The model under review builds one solid part; all positions refer to its coordinate system, in mm. A direction names the side the tool comes from. Round coordinates to 2 decimals unless told otherwise and drop trailing zeros. Order: outer loops, then holes, each group sorted by start corner. A loop starts at its lowest first (then second) coordinate and runs counter-clockwise, first axis right, second up. Notation, with made-up numbers: M -15,73.5 L 44,73.5 A17 ccw 44,80.5 Z; hole C 37,0.5 d11. An arc over 180 degrees is marked long. Use a Markdown table: item, result. Add a question column.
1. The part is to be moulded in two halves that separate along Z. For faces 1 (the flat face through (13, 4, 0)), 2 (the flat face through (0, 5, -12)), 3 (the cylindrical face through (3.451, 3.595, -13.421)), say which applies: +Z half, -Z half, draft (parallel to the pull), parting line (faces both ways), or undercut.
2. Consider section B-B on x = 2.25. State the section outline as (y, z) points.
3. Consider section C-C on y = 5.5. State the section outline as (x, z) points.
4. Insertion check: P1, Ø4, axis at x = 12, y = 4, coming from the -Z side; P2, Ø4, axis at y = 2.75, z = -12.5, coming from the +X side. Each pin has a flat end and moves straight along its axis. Give the tip position at first contact, or say it passes through.
5. Consider section D-D on y = 2.75. State the section outline as (x, z) points, then the cut area to 3 significant figures.
6. For faces 4 (the flat face through (7, 4, -15)), 5 (the flat face through (4, 0, -7)), list the 3-axis set-ups (+Z, -Z, +X, -X, +Y, -Y) from which the entire face can be reached by the end or side of a thin tool; tool diameter is ignored.
7. To check wall thickness, follow probe 1 along Y at (x, z) = (5, -12.5); probe 2 along X at (y, z) = (6.5, -18); probe 3 along Z at (x, y) = (9.25, 0.75). State the ranges of each line that lie inside material, in increasing order.
8. Consider section A-A on z = -22. State the section outline as (x, y) points.
from build123d import *

# Parameters (mm, degrees)
BOSS_EXTRUDE1_DEPTH = 8
CUT_EXTRUDE1_REACH  = 27
SKETCH2_R           = 1.25
CUT_EXTRUDE2_REACH  = 7
SKETCH4_R           = 2.6


with BuildPart() as part:
    # Sketch1 → Boss-Extrude1 (new body)
    with BuildSketch(Plane(origin=(0, 0, 0), x_dir=(1, 0, 0), z_dir=(0, 1, 0))):
        Polygon((0, 0), (0, 25), (7, 25), (7, 5), (25, 5), (25, 0), align=None)
    extrude(amount=BOSS_EXTRUDE1_DEPTH)

    # Sketch2 → Cut-Extrude1 (cut, up to next)
    with BuildSketch(Plane.ZY, mode=Mode.PRIVATE) as cut_extrude1_sk1:
        with Locations((-22, 2.75)):
            Circle(SKETCH2_R)
    cut_extrude1_tool1 = extrude(cut_extrude1_sk1.sketch, amount=-CUT_EXTRUDE1_REACH, mode=Mode.PRIVATE) & part.part
    add(cut_extrude1_tool1.solids().sort_by_distance((0, 2.75, -22))[0], mode=Mode.SUBTRACT)
    # Sketch2 → Cut-Extrude1 (cut, up to next)
    with BuildSketch(Plane.ZY, mode=Mode.PRIVATE) as cut_extrude1_sk2:
        with Locations((-12.5, 2.75)):
            Circle(SKETCH2_R)
    cut_extrude1_tool2 = extrude(cut_extrude1_sk2.sketch, amount=-CUT_EXTRUDE1_REACH, mode=Mode.PRIVATE) & part.part
    add(cut_extrude1_tool2.solids().sort_by_distance((0, 2.75, -12.5))[0], mode=Mode.SUBTRACT)

    # Sketch4 → Cut-Extrude2 (cut, up to next)
    with BuildSketch(Plane(origin=(0, 0, -5), x_dir=(-1, 0, 0), z_dir=(0, 0, -1)), mode=Mode.PRIVATE) as cut_extrude2_sk1:
        with Locations((-17, 4)):
            Circle(SKETCH4_R)
    cut_extrude2_tool1 = extrude(cut_extrude2_sk1.sketch, amount=-CUT_EXTRUDE2_REACH, mode=Mode.PRIVATE) & part.part
    add(cut_extrude2_tool1.solids().sort_by_distance((17, 4, -5))[0], mode=Mode.SUBTRACT)


solid = part.part
Answer block:
| question | item | result |
|---|---|---|
| 1 | face 1 | +Z half |
| 1 | face 2 | draft |
| 1 | face 3 | undercut |
| 2 | outline | M 0,-25 L 8,-25 L 8,0 L 0,0 Z; hole C 2.75,-22 d2.5; hole C 2.75,-12.5 d2.5 |
| 3 | outline | M 0,-25 L 7,-25 L 7,-5 L 14.88,-5 L 14.88,0 L 0,0 Z; M 19.12,-5 L 25,-5 L 25,0 L 19.12,0 Z |
| 4 | P1 | z = -5 |
| 4 | P2 | x = 7 |
| 5 | outline | M 0,-25 L 7,-25 L 7,-23.25 L 0,-23.25 Z; M 0,-20.75 L 7,-20.75 L 7,-13.75 L 0,-13.75 Z; M 0,-11.25 L 7,-11.25 L 7,-5 L 14.72,-5 L 14.72,0 L 0,0 Z; M 19.28,-5 L 25,-5 L 25,0 L 19.28,0 Z |
| 5 | area | 207 mm^2 |
| 6 | face 4 | -Z, +X, +Y, -Y |
| 6 | face 5 | +Z, -Z, +X, -X, -Y |
| 7 | probe 1 | 0 to 1.5, 4 to 8 |
| 7 | probe 2 | 0 to 7 |
| 7 | probe 3 | -5 to 0 |
| 8 | outline | M 0,0 L 7,0 L 7,1.5 L 0,1.5 Z; M 0,4 L 7,4 L 7,8 L 0,8 Z |
